Answer from the drawing. Dimensions are ordinates in mm from the lowest x, y and z of the part. Coordinates: 2 decimals unless noted, no trailing zeros. Loops run counter-clockwise (first coordinate to the right, second up) from the corner with the lowest first, then second, coordinate; pieces in that order, holes last. Notation, with made-up numbers: (12.25, 50.5) - (67.25, 50.5) arc R4 ccw to (67.25, 57.5) - close; hole circle Ø10 at (71, -15). An arc over 180 degrees is marked (long way). Use one line per item in the form item = value. Start each with the question number.
1) The mould has two halves that part along X. Classify the marked faces 1, 2 and 3: released by +X, released by -X, zero draft, split by the parting line, or undercut.
2) A cutting plane is placed at B-B (y = 3.25). Give the vertices of the cut face in (x, z).
3) A cutting plane is placed at C-C (z = 8.25). Give the vertices of the cut face in (x, y).
4) Each of these flat-tipped pins is pushed along its axis until it touches: P1, Ø1, axis at y = 5.5, z = 17.5, coming from the -X side; P2, Ø2, axis at y = 1.5, z = 21, coming from the +X side. Where does it stop, or does it pass through?
5) Consider line 1 (X direction, y = 2.25, z = 16.75); line 2 (X direction, y = 0.75, z = 16.5); line 3 (Z direction, x = 15, y = 5). Determine where each line is inside the solid, lowest interval first.
6) A cutting plane is placed at A-A (x = 41). Give the vertices of the cut face in (y, z).
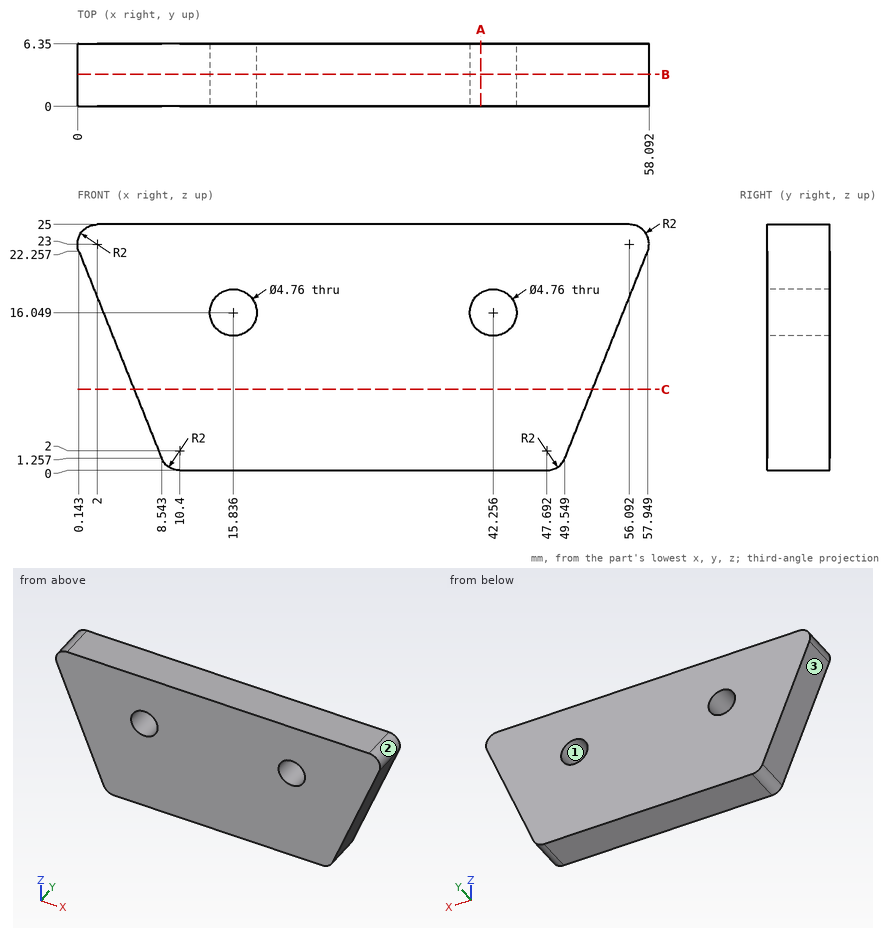
Found:
q1.face_1 = undercut
q1.face_2 = released by +X
q1.face_3 = released by -X
q2.outline = (0.14, 22.26) - (8.54, 1.26) arc R2 ccw to (10.4, 0) - (47.69, 0) arc R2 ccw to (49.55, 1.26) - (57.95, 22.26) arc R2 ccw to (56.09, 25) - (2, 25) arc R2 ccw to start; hole circle Ø4.76 at (15.84, 16.05); hole circle Ø4.76 at (42.26, 16.05)
q3.outline = (5.75, 0) - (52.35, 0) - (52.35, 6.35) - (5.75, 6.35) - close
q4.P1 = 1.85
q4.P2 = 57.85
q5.line_1 = 2.35 to 13.56, 18.11 to 39.98, 44.53 to 55.75
q5.line_2 = 2.45 to 13.5, 18.17 to 39.92, 44.59 to 55.65
q5.line_3 = 0 to 13.82, 18.28 to 25
q6.outline = (0, 0) - (6.35, 0) - (6.35, 14.03) - (0, 14.03) - close; (0, 18.07) - (6.35, 18.07) - (6.35, 25) - (0, 25) - close
